```python
from build123d import *

# Parameters (mm, degrees)
SKETCH1_W           = 50
SKETCH1_H           = 40
BOSS_EXTRUDE1_DEPTH = 10
SKETCH5_W           = 6
SKETCH5_H           = 5
BOSS_EXTRUDE3_DEPTH = 10
SKETCH6_R           = 2
CUT_EXTRUDE1_DEPTH  = 20
SKETCH8_W           = 10
SKETCH8_H           = 40
CUT_EXTRUDE2_DEPTH  = 25
SKETCH9_W           = 10
SKETCH9_H           = 6
SKETCH9_R           = 1.930897171
BOSS_EXTRUDE4_DEPTH = 5
SKETCH10_W          = 10
SKETCH10_H          = 5
CUT_EXTRUDE3_DEPTH  = 15
SKETCH11_W          = 5
SKETCH11_H          = 5
BOSS_EXTRUDE5_DEPTH = 10
SKETCH12_R          = 1.5
CUT_EXTRUDE4_DEPTH  = 10


with BuildPart() as part:
    # Sketch1 → Boss-Extrude1 (new body)
    with BuildSketch(Plane(origin=(669.84184187, 0, 0), x_dir=(1, 0, 0), z_dir=(0, 0, 1))):
        with Locations((-671.310344828, 437.637931034)):
            Rectangle(SKETCH1_W, SKETCH1_H)
    boss_extrude1 = extrude(amount=BOSS_EXTRUDE1_DEPTH)

    # Sketch5 → Boss-Extrude3 (add)
    with BuildSketch(Plane(origin=(23.531497042, 0, 0), x_dir=(0, 0, -1), z_dir=(1, 0, 0))):
        with Locations((-5, 442.637931034)):
            Rectangle(SKETCH5_W, SKETCH5_H)
        with Locations((-5, 432.637931034)):
            Rectangle(SKETCH5_W, SKETCH5_H)
    extrude(amount=BOSS_EXTRUDE3_DEPTH)

    # Sketch6 → Cut-Extrude1 (cut)
    with BuildSketch(Plane(origin=(669.84184187, 445.137931034, 0), x_dir=(1, 0, 0), z_dir=(0, 1, 0))):
        with Locations(Location((-641.310344828, -5, 0), (0, 0, 180))):
            Circle(SKETCH6_R)
    extrude(amount=-CUT_EXTRUDE1_DEPTH, mode=Mode.SUBTRACT)

    # Sketch8 → Cut-Extrude2 (cut)
    with BuildSketch(Plane.ZY.offset(26.468502958)):
        with Locations((5, 437.637931034)):
            Rectangle(SKETCH8_W, SKETCH8_H)
    extrude(amount=-CUT_EXTRUDE2_DEPTH, mode=Mode.SUBTRACT)

    # Sketch9 → Boss-Extrude4 (add)
    with BuildSketch(Plane(origin=(0, 435.137931034, 0), x_dir=(1, 0, 0), z_dir=(0, 1, 0))):
        with Locations((28.531497042, -5)):
            Rectangle(SKETCH9_W, SKETCH9_H)
        with Locations(Location((28.531497042, -5, 0), (0, 0, 180))):
            Circle(SKETCH9_R, mode=Mode.SUBTRACT)
    extrude(amount=BOSS_EXTRUDE4_DEPTH)

    # Sketch10 → Cut-Extrude3 (cut)
    with BuildSketch(Plane.XY.offset(8)):
        with Locations((28.531497042, 432.637931034)):
            Rectangle(SKETCH10_W, SKETCH10_H)
        with Locations((28.531497042, 442.637931034)):
            Rectangle(SKETCH10_W, SKETCH10_H)
    extrude(amount=-CUT_EXTRUDE3_DEPTH, mode=Mode.SUBTRACT)

    # Mirror1: Boss-Extrude1 across plane
    add(boss_extrude1.mirror(Plane(origin=(-1.468502958, 0, 0), x_dir=(0, 0, 1), z_dir=(1, 0, 0))))

    # Sketch11 → Boss-Extrude5 (add)
    with BuildSketch(Plane(origin=(0, 457.637931034, 0), x_dir=(1, 0, 0), z_dir=(0, 1, 0))):
        with Locations((-1.468502958, -5)):
            Rectangle(SKETCH11_W, SKETCH11_H)
    extrude(amount=BOSS_EXTRUDE5_DEPTH)

    # Sketch12 → Cut-Extrude4 (cut)
    with BuildSketch(Plane(origin=(1.031497042, 0, 0), x_dir=(0, 0, -1), z_dir=(1, 0, 0))):
        with Locations((-5, 462.637931034)):
            Circle(SKETCH12_R)
    extrude(amount=-CUT_EXTRUDE4_DEPTH, mode=Mode.SUBTRACT)


solid = part.part
```
The model under review builds one solid part; all positions refer to its coordinate system, in mm. A direction names the side the tool comes from. Round coordinates to 2 decimals unless told otherwise and drop trailing zeros. Order: outer loops, then holes, each group sorted by start corner. A loop starts at its lowest first (then second) coordinate and runs counter-clockwise, first axis right, second up. Notation, with made-up numbers: M 81,56 L 107,56 A11 ccw 107,69 Z; hole C -2,16 d3. An arc over 180 degrees is marked long. Use a Markdown table: item, result.
1) Consider section A-A (z = 5). Write out the cut boundary in (x, y), then the cut area to 3 significant figures.
Report:
| item | result |
|---|---|
| outline | M -26.47,417.64 L 23.53,417.64 L 23.53,435.14 L 26.6,435.14 L 26.6,440.14 L 23.53,440.14 L 23.53,457.64 L 1.03,457.64 L 1.03,461.14 L -3.97,461.14 L -3.97,457.64 L -26.47,457.64 Z; M -3.97,464.14 L 1.03,464.14 L 1.03,467.64 L -3.97,467.64 Z; M 30.46,435.14 L 33.53,435.14 L 33.53,440.14 L 30.46,440.14 Z |
| area | 2,070 mm^2 |
2) Wall thickness on line 1 along Y through (x, z) = (-1.1, 5); line 2 along Y through (x, z) = (7.5, 8); line 3 along Z through (x, y) = (30, 436.5): over which ranges is each line inside the solid? List them lowest first. Write a range as [from, to].
Report:
| item | result |
|---|---|
| line 1 | [417.64, 461.14], [464.14, 467.64] |
| line 2 | [417.64, 457.64] |
| line 3 | [2, 3.75], [6.25, 8] |
3) Tool access review of faces 1 (the face through (28, 438, 8)), 2 (the face through (26, 435.138, 5)), 3 (the face through (1.031, 461, 6)), 4 (the face through (28, 438, 2)), 5 (the face through (-3.969, 461, 6)): name each direction out of +Z, -Z, +X, -X, +Y, -Y from which nothing blocks a thin tool from reaching the whole face with its end or side.
Report:
| item | result |
|---|---|
| face 1 | +Z, +X, +Y, -Y |
| face 2 | +Z, -Z, +X, -Y |
| face 3 | +Z, -Z, +X, +Y |
| face 4 | -Z, +X, +Y, -Y |
| face 5 | +Z, -Z, -X, +Y |
4) Consider section C-C (y = 432). Write out the cut boundary in (x, z).
Report:
| item | result |
|---|---|
| outline | M -26.47,0 L 23.53,0 L 23.53,10 L -26.47,10 Z |
5) Insertion check: pin 1 (1.5 mm diameter, centred on y = 460.5, z = 6, fed in from -X); pin 2 (6 mm diameter, centred on x = 5.5, y = 427.5, fed in from -Z); pin 3 (5.5 mm diameter, centred on x = 30, y = 438, fed in from -Z); pin 4 (2 mm diameter, centred on x = 26, y = 454.5, fed in from -Z). Each pin has a flat end and moves straight along its axis. Give the tip position at first contact, or say it passes through.
Report:
| item | result |
|---|---|
| pin 1 | x = -3.97 |
| pin 2 | z = 0 |
| pin 3 | z = 2 |
| pin 4 | through |
6) Consider section D-D (x = 6). Write out the cut boundary in (y, z), then the cut area to 3 significant figures.
Report:
| item | result |
|---|---|
| outline | M 417.64,0 L 457.64,0 L 457.64,10 L 417.64,10 Z |
| area | 400 mm^2 |
7) Draft analysis for pull direction Z (two halves, no side actions). For faces 6 (the face through (-1.434, 461.307, 4.308)), 7 (the face through (-2, 463, 2.5)), 8 (the face through (-26.469, 437, 5)), state which applies: released by +Z, released by -Z, zero draft, split by the parting line, or undercut.
Report:
| item | result |
|---|---|
| face 6 | undercut |
| face 7 | released by -Z |
| face 8 | zero draft |
8) Consider section B-B (x = -1.5). Write out the cut boundary in (y, z).
Report:
| item | result |
|---|---|
| outline | M 417.64,0 L 457.64,0 L 457.64,2.5 L 467.64,2.5 L 467.64,7.5 L 457.64,7.5 L 457.64,10 L 417.64,10 Z; hole C 462.64,5 d3 |
